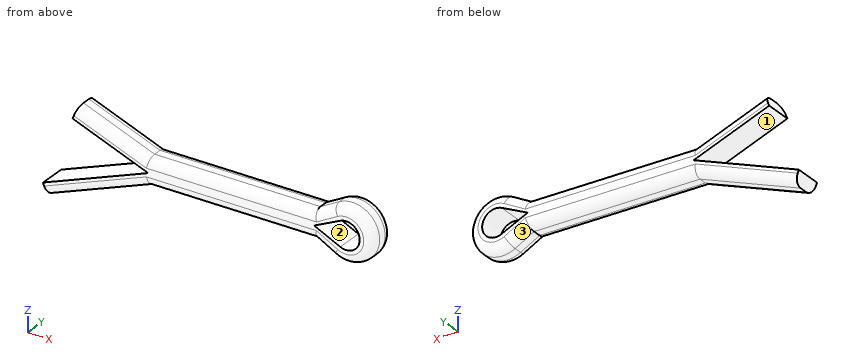
Autodesk Inventor part; units mm, degrees
ref_plane "Work Plane1" through (0, -10, 0) normal (0, 0, -1) x (0, 1, 0)
ref_plane "Work Plane3" through (0, 0, 1.15) normal (-1, 0, 0) x (0, 1, 0)
ref_plane "YZ Plane" through (0, 0, 0) normal (1, 0, 0) x (0, 1, 0)
sketch "Sketch1" plane through (0, 0, 0) normal (0, 1, 0) x (-1, 0, 0)
  arc A0 (-1.6014, 2.0207) -> (-1.6014, -2.0207) centre (-2.7, 0) ccw
  arc A1 (-2.2102, 1.0405) -> (-2.2102, -1.0405) centre (-2.7, 0) ccw
  line L0 (0, 1.15) -> (14, 1.15)
  line L1 (0, -1.15) -> (14, -1.15)
  line L2 (14, 1.15) -> (20, 3.4487)
  line L3 (20, 3.4487) -> (20.3842, 2.4459)
  line L4 (20.3842, 2.4459) -> (14, 0)
  line L5 (14, 0) -> (22.8842, -3.4037)
  line L6 (22.8842, -3.4037) -> (22.5, -4.4065)
  line L7 (22.5, -4.4065) -> (14, -1.15)
  line L8 (0, 0) -> (-2.2102, -1.0405)
  line L9 (0, 0) -> (-2.2102, 1.0405)
  line L10 (0, 1.15) -> (0, -1.15) construction
  line L11 (0, 1.15) -> (-1.6014, 2.0207)
  line L12 (0, -1.15) -> (-1.6014, -2.0207)
  line L13 (-5, 0) -> (14, 0) construction
  line L14 (14, 1.15) -> (14, -1.15) construction
  dimension "d0" = 14
  dimension "d1" = 20
  dimension "d2" = 159.037
  dimension "d3" = 159.037
  dimension "d4" = 2.5
  dimension "d5" = 1.15
  dimension "d6" = 2.3
  dimension "d7" = 1.15
  dimension "d8" = 1.15
  dimension "d9" = 2.7
extrude "Body" add sketch "Sketch1" along normal mid plane 2.3
fillet "Fillet" radius 0.805 14 edges at (-17, -1.15, 2.2994) (-17, 1.15, 2.2994) (-7, -1.15, 1.15) (-7, 1.15, 1.15) (5, -1.15, 0) (0.8007, -1.15, -1.5853) (0.8007, -1.15, 1.5853) (5, 1.15, 0) (0.8007, 1.15, 1.5853) (0.8007, 1.15, -1.5853) (-7, -1.15, -1.15) (-18.25, -1.15, -2.7783) (-7, 1.15, -1.15) (-18.25, 1.15, -2.7783)
ref_plane "Work Plane1" through (0, -10, 0) normal (0, 0, -1) x (0, 1, 0)
ref_plane "Work Plane3" through (0, 0, 1.15) normal (-1, 0, 0) x (0, 1, 0)
equation "\"d0\" = MSIAB"
equation "\"d1\" = SNLG"
equation "\"d4\" = LGDIF"
equation "\"d5\" = -0.5 * SNND1 + 0.5 * KBR"
equation "\"d6\" = 0.5 * KBR"
equation "\"d7\" = 0.5 * SNND1"
equation "\"d8\" = 0.5 * SNND1"
equation "\"d9\" = KOL - 0.5 * KBR"
equation "\"d10\" = SNND1"
equation "\"d12\" = 0.35 * SNND1"
equation "\"SNND\" = 2.5"
equation "\"SNLG\" = 20"
equation "\"SNND1\" = 2.3"
equation "\"KBR\" = 4.6"
equation "\"KOL\" = 5"
equation "\"LGDIF\" = 2.5"
equation "\"MSIAB\" = 14"
equation "\"NNDMAX\" = 11"
equation "\"DSH\" = 5"
equation "\"NNDMIN\" = 9"
properties part number "100003" material "Steel, Mild"
Build history of the part. All positions in model axes, mm. Face numbers are marked on the shaded views. Round coordinates to 2 decimals unless told otherwise and drop trailing zeros. Write each loop counter-clockwise with the first axis right and the second up, starting at its lowest first coordinate (ties: lowest second). Pieces come first, ordered by that corner, then holes. Notation, with made-up numbers: (18, 10) -> (53, 10) arc R19 cw to (53, 43) -> close; hole circle Ø9 at (32, 74.5). An arc over 180 degrees is marked (long way). Use one line per item in the form item = value.
Q1. Drill centre lines: L1, parallel to Z at x = 2.7, y = 0; L2, parallel to Z at x = 1.25, y = 0.55; L3, parallel to Y at x = -2.5, z = -0.75. Where is each one in solid material? Low to high.
Conclusion:
L1 = -2.3 to -1.15, 1.15 to 2.3
L2 = -1.8 to -0.59, 0.59 to 1.8
L3 = -1.04 to 1.04
Q2. Band-saw the part on C-C, the plane x = -9.5. Write the cut outline in (y, z) (3 decimals), then the cut area to 3 significant figures.
Conclusion:
outline = (-1.15, -0.345) arc R0.805 ccw to (-0.345, -1.15) -> (0.345, -1.15) arc R0.805 ccw to (1.15, -0.345) -> (1.15, 0.345) arc R0.805 ccw to (0.345, 1.15) -> (-0.345, 1.15) arc R0.805 ccw to (-1.15, 0.345) -> close
area = 4.73 mm²
Q3. Two-plate mould, pull along Z, no slides. Class the marked faces 1, 2 and 3: released by +Z, released by -Z, zero draft, split by the parting line, or undercut.
Conclusion:
face_1 = undercut
face_2 = undercut
face_3 = released by -Z
Q4. Band-saw the part on A-A, the plane x = 2.7. Write the cut outline in (y, z) (3 decimals), then the cut area to 3 significant figures.
Conclusion:
outline = (-1.15, -1.495) arc R0.805 ccw to (-0.345, -2.3) -> (0.345, -2.3) arc R0.805 ccw to (1.15, -1.495) -> (1.15, -1.15) -> (-1.15, -1.15) -> close; (-1.15, 1.15) -> (1.15, 1.15) -> (1.15, 1.495) arc R0.805 ccw to (0.345, 2.3) -> (-0.345, 2.3) arc R0.805 ccw to (-1.15, 1.495) -> close
area = 4.73 mm²
Q5. Band-saw the part on B-B, the plane y = 0. Write the cut outline in (x, z), then the cut area to 3 significant figures.
Conclusion:
outline = (-22.88, -3.4) -> (-22.5, -4.41) -> (-14, -1.15) -> (0, -1.15) -> (1.6, -2.02) arc R2.3 ccw (long way) to (1.6, 2.02) -> (0, 1.15) -> (-14, 1.15) -> (-20, 3.45) -> (-20.38, 2.45) -> (-14, 0) -> close; hole (0, 0) -> (2.21, -1.04) arc R1.15 ccw (long way) to (2.21, 1.04) -> close
area = 62.1 mm²
Q6. Drop a flat-ended pin along its axis: P1, Ø0.8, axis at x = -4, y = 0, coming from the -Z side. Give the stop position or say it passes through.
Conclusion:
P1 = -1.15
